The model under review builds one solid part; all positions refer to its coordinate system, in mm. Face numbers are marked on the shaded views. Round coordinates to 2 decimals unless told otherwise and drop trailing zeros. Order: outer loops, then holes, each group sorted by start corner. A loop starts at its lowest first (then second) coordinate and runs counter-clockwise, first axis right, second up. Notation, with made-up numbers: M 72.5,32.25 L 80.5,32.25 A31 ccw 80.5,56.25 Z; hole C 70,-39.75 d2. An arc over 180 degrees is marked long. Answer as a JSON object with one key per item and string values. Group by question number.
1. Mouldability with a two-part tool opening along Z and no side actions: class the marked faces 1 and 2 as released by +Z, released by -Z, zero draft, split by the parting line, or undercut.
2. Add section B-B on x = 0. State the section outline as (y, z) points.
3. To check wall thickness, follow probe 1 along Y at (x, z) = (0.25, 25); probe 2 along X at (y, z) = (-2, 9). State the ranges of each line that lie inside material, in increasing order. Write a range as [from, to].
4. Add section A-A on y = -6. State the section outline as (x, z) points, and give its area (3 significant figures).
5. Add section D-D on x = -3.75. State the section outline as (y, z) points.
6. Add section C-C on z = 19.75. State the section outline as (x, y) points, and give its area (3 significant figures).
7. Clearance check with flat-ended pins moving along their axes: P1, Ø0.8, axis at x = 0.5, z = 9, coming from the -Y side; P2, Ø2, axis at x = 3, y = -2, coming from the +Z side; P3, Ø5, axis at y = -6, z = 11.5, coming from the -X side. State where each tip first meets the part, or that it passes through.
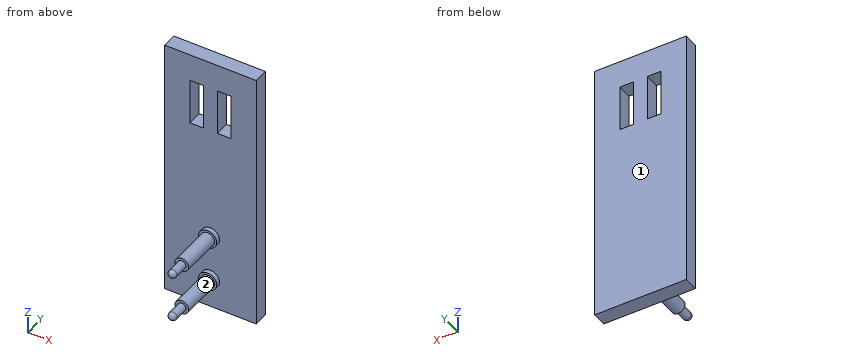
```python
from build123d import *

# Parameters (mm, degrees)
SKETCH1_W           = 10
SKETCH1_H           = 31.69
SKETCH1_W_2         = 1.5
SKETCH1_H_2         = 5
BOSS_EXTRUDE1_DEPTH = 1.6
SKETCH4_R           = 1
BOSS_EXTRUDE2_DEPTH = 0.5
SKETCH5_R           = 0.75
BOSS_EXTRUDE3_DEPTH = 4.5
SKETCH6_R           = 0.45
BOSS_EXTRUDE4_DEPTH = 2
FILLET1_R           = 0.45
SKETCH7_W           = 10
SKETCH7_H           = 3
CUT_EXTRUDE1_DEPTH  = 10


with BuildPart() as part:
    # Sketch1 → Boss-Extrude1 (new body)
    with BuildSketch(Plane(origin=(0, 0, 0), x_dir=(1, 0, 0), z_dir=(0, 1, 0))):
        with Locations((0, -21.731751346)):
            Rectangle(SKETCH1_W, SKETCH1_H)
        with Locations((1.5, -29.076751346)):
            Rectangle(SKETCH1_W_2, SKETCH1_H_2, mode=Mode.SUBTRACT)
        with Locations((-1.5, -29.076751346)):
            Rectangle(SKETCH1_W_2, SKETCH1_H_2, mode=Mode.SUBTRACT)
    extrude(amount=BOSS_EXTRUDE1_DEPTH)

    # Sketch4 → Boss-Extrude2 (add)
    with BuildSketch(Plane.XZ):
        with Locations(Location((0, 9.136751346, 0), (0, 0, 90))):
            Circle(SKETCH4_R)
        with Locations(Location((0, 14.136751346, 0), (0, 0, 90))):
            Circle(SKETCH4_R)
    extrude(amount=BOSS_EXTRUDE2_DEPTH)

    # Sketch5 → Boss-Extrude3 (add)
    with BuildSketch(Plane.XZ.offset(0.5)):
        with Locations(Location((0, 9.136751346, 0), (0, 0, 270))):
            Circle(SKETCH5_R)
        with Locations(Location((0, 14.136751346, 0), (0, 0, 270))):
            Circle(SKETCH5_R)
    extrude(amount=BOSS_EXTRUDE3_DEPTH)

    # Sketch6 → Boss-Extrude4 (add)
    with BuildSketch(Plane.XZ.offset(5)):
        with Locations(Location((0, 9.136751346, 0), (0, 0, 270))):
            Circle(SKETCH6_R)
        with Locations(Location((0, 14.136751346, 0), (0, 0, 270))):
            Circle(SKETCH6_R)
    extrude(amount=BOSS_EXTRUDE4_DEPTH)

    # Fillet1
    fillet1_edges = [part.edges().sort_by_distance(p)[0] for p in [
        (0, -7, 9.586751346),
        (0, -7, 14.586751346),
    ]]
    fillet(fillet1_edges, radius=FILLET1_R)

    # Sketch7 → Cut-Extrude1 (cut)
    with BuildSketch(Plane.XZ):
        with Locations((0, 36.076751346)):
            Rectangle(SKETCH7_W, SKETCH7_H)
    extrude(amount=-CUT_EXTRUDE1_DEPTH, mode=Mode.SUBTRACT)


solid = part.part
```
Recorded:
{
 "1": {"face 1": "zero draft", "face 2": "undercut"},
 "2": {"outline": "M -6.55,8.69 L -5,8.69 L -5,8.39 L -0.5,8.39 L -0.5,8.14 L 0,8.14 L 0,5.89 L 1.6,5.89 L 1.6,34.58 L 0,34.58 L 0,15.14 L -0.5,15.14 L -0.5,14.89 L -5,14.89 L -5,14.59 L -6.55,14.59 A0.45 ccw -6.55,13.69 L -5,13.69 L -5,13.39 L -0.5,13.39 L -0.5,13.14 L 0,13.14 L 0,10.14 L -0.5,10.14 L -0.5,9.89 L -5,9.89 L -5,9.59 L -6.55,9.59 A0.45 ccw Z"},
 "3": {"probe 1": "y = [0, 1.6]", "probe 2": "x = [-0.74, 0.74]"},
 "4": {"outline": "C 0,9.14 d0.9; C 0,14.14 d0.9", "area": "1.27 mm²"},
 "5": {"outline": "M 0,5.89 L 1.6,5.89 L 1.6,34.58 L 0,34.58 Z"},
 "6": {"outline": "M -5,0 L 5,0 L 5,1.6 L -5,1.6 Z", "area": "16.0 mm²"},
 "7": {"P1": "stops at y = -6.98", "P2": "passes through", "P3": "stops at x = -0.75"}
}
